```python
from build123d import *

# Parameters (mm, degrees)
F1_DEPTH = 165.1
F2_W     = 304.8
F2_H     = 63.5
F3_DEPTH = 330.2


with BuildPart() as f1:
    # F0 (on Front) → F1 (new body, symmetric)
    with BuildSketch(Plane.XZ):
        Polygon((0, 342.9), (0, 0), (0, -63.5), (63.5, -63.5), (63.5, 342.9), align=None)
    extrude(amount=F1_DEPTH, both=True)

    # F2 (on face) → F3 (join)
    with BuildSketch(Plane.XZ.offset(165.1)):
        with Locations((-152.4, -31.75)):
            Rectangle(F2_W, F2_H)
    extrude(amount=-F3_DEPTH)


solid = f1.part
```
The listing builds one solid part. Answer for the finished solid, in the listing's coordinates (mm). A direction names the side the tool comes from. Round coordinates to 2 decimals unless told otherwise and drop trailing zeros. Loops run counter-clockwise (first coordinate to the right, second up) from the corner with the lowest first, then second, coordinate; pieces in that order, holes last. Notation, with made-up numbers: (24.5, -14.75) - (45.5, -14.75) arc R4 ccw to (45.5, -9.75) - close; hole circle Ø10 at (76, -23). An arc over 180 degrees is marked (long way). Use one line per item in the form item = value. Start each with the question number.
1. The part is cut by section C-C on z = 128. Determine the outline of the cut face in (x, y), then the cut area to 3 significant figures.
2. Given pin 1 Ø3 at (y, z) = (115, 285) entering from -X, flat-ended and moving along its own axis, determine where the tip first touches the part or whether it passes through.
3. Consider line 1 (Z direction, x = -177, y = 141.5); line 2 (X direction, y = 29, z = 293.5). Determine where each line is inside the solid, lowest interval first. Write a range as [from, to].
4. The part is cut by section B-B on y = -107.5. Determine the outline of the cut face in (x, z), then the cut area to 3 significant figures.
5. The part is cut by section A-A on x = -130. Determine the outline of the cut face in (y, z).
6. A tool of negligible diameter and unlimited length cuts with its end or side. For faces 1 (the face through (-155, -2, 0)), 2 (the face through (-123, -2, -63.5)), from which of +Z, -Z, +X, -X, +Y, -Y can it reach the whole face along a straight path? Write none if from no direction.
Geometry check:
q1.outline = (0, -165.1) - (63.5, -165.1) - (63.5, 165.1) - (0, 165.1) - close
q1.area = 21,000 mm^2
q2.pin_1 = 0
q3.line_1 = [-63.5, 0]
q3.line_2 = [0, 63.5]
q4.outline = (-304.8, -63.5) - (63.5, -63.5) - (63.5, 342.9) - (0, 342.9) - (0, 0) - (-304.8, 0) - close
q4.area = 45,200 mm^2
q5.outline = (-165.1, -63.5) - (165.1, -63.5) - (165.1, 0) - (-165.1, 0) - close
q6.face_1 = +Z, -X, +Y, -Y
q6.face_2 = -Z, +X, -X, +Y, -Y
